```python
from build123d import *

# Parameters (mm, degrees)
F0_W     = 30
F0_H     = 5
F0_R     = 1
F1_DEPTH = 3
F2_DEPTH = 6.95745
F4_W     = 0.5
F4_H     = 4.2


with BuildPart() as f1:
    # F0 (on Front) → F1 (new body)
    with BuildSketch(Plane.XZ):
        Rectangle(F0_W, F0_H)
        Circle(F0_R, mode=Mode.SUBTRACT)
    extrude(amount=F1_DEPTH)

    # F0 (on Front) → F2 (join)
    with BuildSketch(Plane.XZ):
        Circle(F0_R)
    extrude(amount=F2_DEPTH)

    # F5: sweep along a path in F3
    with BuildLine(Plane.XY) as f5_path:
        Line((-7.035956, 7.03008), (0, 0))
    # F4 (on face) → F5 (sweep)
    with BuildSketch(Plane(origin=(0, 0, 0), x_dir=(-1, 0, 0), z_dir=(0, 1, 0))):
        Rectangle(F4_W, F4_H)
    sweep(path=f5_path.line)

    # F6: sweep along a path in F3
    with BuildLine(Plane.XY) as f6_path:
        Line((7.035956, 7.03008), (0, 0))
    # F4 (on face) → F6 (sweep)
    with BuildSketch(Plane(origin=(0, 0, 0), x_dir=(-1, 0, 0), z_dir=(0, 1, 0))):
        Rectangle(F4_W, F4_H)
    sweep(path=f6_path.line)


solid = f1.part
```
Source: CAD feature listing. Evaluate the final solid. Frame: model axes, mm. A direction names the side the tool comes from. Give positions to 0.01 mm unless a question says otherwise; leave off trailing zeros. Loops run counter-clockwise (first coordinate to the right, second up) from the corner with the lowest first, then second, coordinate; pieces in that order, holes last. Notation, with made-up numbers: (32, 75.25) -> (69, 75.25) arc R9 cw to (69, 80.25) -> close; hole circle Ø4 at (26.5, 40.25). An arc over 180 degrees is marked (long way). Put each result on its own line as item: value. Start each with the question number.
1) Material intervals for probe 1 along Y at (x, z) = (7.5, -1.75); probe 2 along X at (y, z) = (4.25, 1.4); probe 3 along Y at (x, z) = (6.75, -1.1), sorted ascending.
2) Cut plane B-B (x = 3.25). Return loops of the section in (y, z).
3) Reachability of faces 4 (the face through (3.345, 3.592, -0.029)), 5 (the face through (0, -5, -1)), 6 (the face through (2, 2, -2.1)), 7 (the face through (-2, 2, 2.1)) from +Z, -Z, +X, -X, +Y, -Y: full face, straight path, thin tool, end or side. Return the list, or none.
4) Cut plane A-A (z = 0). Return loops of the section in (x, y).
5) Cut plane C-C (y = -4.5). Return loops of the section in (x, z), then the cut area to 3 significant figures.
6) Cut plane D-D (x = -12.25). Return loops of the section in (y, z), then the cut area to 3 significant figures.
7) Draft query along Y for faces 1 (the face through (3.719, 3.466, 0.029)), 2 (the face through (-3.345, 3.592, 0.029)), 3 (the face through (15, -1, 0)). Return one class per face: released by +Y, released by -Y, zero draft, split by the parting line, or undercut.
8) Contact query for flat-ended pins moving along their axis: P1, Ø2, axis at y = -5.5, z = -0.5, coming from the +X side; P2, Ø2.5, axis at x = 5, z = 1, coming from the +Y side; P3, Ø3.5, axis at x = -1.5, y = 3, coming from the +Z side. Output: stop coordinate, or through.
Results are:
1. probe 1: y = -3 to 0
1. probe 2: x = -4.5 to -4, 4 to 4.5
1. probe 3: y = -3 to 0, 6.49 to 6.99
2. outline: (-3, -2.5) -> (0, -2.5) -> (0, 2.5) -> (-3, 2.5) -> close; (3, -2.1) -> (3.5, -2.1) -> (3.5, 2.1) -> (3, 2.1) -> close
3. face 4: +Z, -Z, +Y
3. face 5: -Y
3. face 6: -Z, +X, -X, +Y
3. face 7: +Z, +X, -X, +Y
4. outline: (-15, -3) -> (-1, -3) -> (-1, -6.96) -> (1, -6.96) -> (1, -3) -> (15, -3) -> (15, 0) -> (0.25, 0) -> (7.29, 7.03) -> (6.79, 7.03) -> (0, 0.25) -> (-6.79, 7.03) -> (-7.29, 7.03) -> (-0.25, 0) -> (-15, 0) -> close
5. outline: circle Ø2 at (0, 0)
5. area: 3.14 mm2
6. outline: (-3, -2.5) -> (0, -2.5) -> (0, 2.5) -> (-3, 2.5) -> close
6. area: 15.0 mm2
7. face 1: undercut
7. face 2: released by +Y
7. face 3: zero draft
8. P1: stops at x = 1
8. P2: stops at y = 6.49
8. P3: stops at z = 2.1
